Geometry: final body of the model. Coordinates: model frame, mm. A direction names the side the tool comes from. Give positions to 0.01 mm unless a question says otherwise; leave off trailing zeros. Write each loop counter-clockwise with the first axis right and the second up, starting at its lowest first coordinate (ties: lowest second). Pieces come first, ordered by that corner, then holes. Notation, with made-up numbers: (-13.75, 84) - (40.25, 84) arc R16 ccw to (40.25, 114) - close; hole circle Ø6 at (44.25, 9.25). An arc over 180 degrees is marked (long way). Use CSV: the item, a comma, the result in double quotes. Start each with the question number.
(1) Section B-B on z = -99. Output: boundary loops of the cut face in (x, y).
(2) Section D-D on y = 62. Output: boundary loops of the cut face in (x, z).
(3) Reachability of faces 1 (the flat face through (-14, -14.263, -60)), 2 (the flat face through (100, -10, 3)), 3 (the flat face through (-13, 48, -127)), 4 (the flat face through (46.2, 123.5, -39.49)) from +Z, -Z, +X, -X, +Y, -Y: full face, straight path, thin tool, end or side. Return the list, or none.
(4) Line query: probe 1 along Y at (x, z) = (-13, -113); probe 2 along X at (y, z) = (69.5, -67); probe 3 along X at (y, z) = (36, 0). Output: solid intervals per line, ascending. Write a range as [from, to].
(5) First-contact query: pin 1 Ø12 at (x, z) = (97.5, -53) entering from -Y; pin 2 Ø7.5 at (x, y) = (-12, -26.5) entering from -Z; pin 3 Ø3 at (y, z) = (55.5, -126) entering from +X. Flat tips, straight axial feed; report the tip coordinate or a pass-through.
(6) Section A-A on x = 41.5. Output: boundary loops of the cut face in (y, z).
(7) Draft query along X for faces 5 (the cylindrical face through (-13.55, 112.16, -41.09)), 6 (the flat face through (65, -10, 3)), 7 (the flat face through (-2.5, 76, -18)), 8 (the flat face through (105, -10, 3)). Return one class per face: released by +X, released by -X, zero draft, split by the parting line, or undercut.
(8) Section C-C on z = -21. Output: boundary loops of the cut face in (x, y), and give its area (3 significant figures).
from build123d import *

# Parameters (mm, degrees)
SKETCH1_W                = 170
SKETCH1_H                = 130
BOSS_EXTRUDE1_DEPTH      = 8
SKETCH2_R                = 1.5
SKETCH2_W                = 165
SKETCH2_H                = 100
CUT_EXTRUDE1_DEPTH       = 21
SKETCH3_W                = 170
SKETCH3_H                = 20
BOSS_EXTRUDE2_DEPTH      = 8
SKETCH4_W                = 65
SKETCH4_H                = 16.2
CUT_EXTRUDE2_DEPTH       = 2
SKETCH5_W                = 3.5
SKETCH5_H                = 12
CUT_EXTRUDE3_DEPTH       = 35
SKETCH6_W                = 170
SKETCH6_H                = 150
BOSS_EXTRUDE3_DEPTH      = 8
BOSS_EXTRUDE4_DEPTH      = 138
SKETCH8_W                = 249
SKETCH8_H                = 138
BOSS_EXTRUDE5_DEPTH      = 1
SKETCH9_W                = 72.8
SKETCH9_H                = 73.25
CUT_EXTRUDE4_DEPTH       = 19
BOSS_EXTRUDE6_DEPTH      = 5
SKETCH11_R               = 1.5
CUT_EXTRUDE5_DEPTH       = 56
SKETCH12_R               = 9
SKETCH12_R_2             = 6.5
SKETCH12_R_3             = 1
SKETCH12_R_4             = 2.75
CUT_EXTRUDE6_DEPTH       = 115
SKETCH13_W               = 58.59049163
SKETCH13_H               = 30.075830986
CUT_EXTRUDE7_DEPTH       = 3
FILLET1_R                = 2
SKETCH15_R               = 1.5
CUT_EXTRUDE8_DEPTH       = 10
CUT_EXTRUDE10_DEPTH      = 261
SKETCH19_R               = 1.5
BOSS_EXTRUDE7_DEPTH      = 8
BOSS_EXTRUDE12_START     = -124.5
BOSS_EXTRUDE12_DEPTH     = 249
SKETCH22_R               = 1.5
SKETCH22_W               = 165
SKETCH22_H               = 100
CUT_EXTRUDE11_DEPTH      = 18
FILLET2_R                = 10
SKETCH24_R               = 2
SKETCH24_W               = 3
SKETCH24_H               = 72
CUT_EXTRUDE15_DEPTH      = 42
CUT_EXTRUDE16_DEPTH      = 140
CUT_EXTRUDE16_DEPTH_BACK = 242
SKETCH27_W               = 249
SKETCH27_H               = 105
BOSS_EXTRUDE13_DEPTH     = 7
CUT_EXTRUDE17_DEPTH      = 249
FILLET6_R                = 3
FILLET7_R                = 3
BOSS_EXTRUDE14_DEPTH     = 9
SKETCH30_R               = 1.5
CUT_EXTRUDE18_DEPTH      = 10
SKETCH31_R               = 1.5
CUT_EXTRUDE19_DEPTH      = 49
CUT_EXTRUDE20_DEPTH      = 49
SKETCH33_W               = 129
SKETCH33_H               = 190
CUT_EXTRUDE21_DEPTH      = 200


with BuildPart() as part:
    # Sketch1 → Boss-Extrude1 (new body)
    with BuildSketch(Plane.XY):
        with Locations((85, 65)):
            Rectangle(SKETCH1_W, SKETCH1_H)
    extrude(amount=BOSS_EXTRUDE1_DEPTH)

    # Sketch2 → Cut-Extrude1 (cut)
    with BuildSketch(Plane.XY.offset(8)):
        with Locations((6.55, 123.35)):
            Circle(SKETCH2_R)
        with Locations((163.45, 123.35)):
            Circle(SKETCH2_R)
        with Locations((6.55, 6.65)):
            Circle(SKETCH2_R)
        with Locations((163.45, 6.65)):
            Circle(SKETCH2_R)
        with Locations((85, 65)):
            Rectangle(SKETCH2_W, SKETCH2_H)
    extrude(amount=-CUT_EXTRUDE1_DEPTH, mode=Mode.SUBTRACT)

    # Sketch3 → Boss-Extrude2 (add)
    with BuildSketch(Plane.XY.offset(8)):
        with Locations((85, -10)):
            Rectangle(SKETCH3_W, SKETCH3_H)
    extrude(amount=-BOSS_EXTRUDE2_DEPTH)

    # Sketch4 → Cut-Extrude2 (cut)
    with BuildSketch(Plane.XY.offset(8)):
        with Locations((85, -10)):
            Rectangle(SKETCH4_W, SKETCH4_H)
    extrude(amount=-CUT_EXTRUDE2_DEPTH, mode=Mode.SUBTRACT)

    # Sketch5 → Cut-Extrude3 (cut)
    with BuildSketch(Plane.XY.offset(6)):
        with Locations((63.25, -10)):
            Rectangle(SKETCH5_W, SKETCH5_H)
        with Locations((71.75, -10)):
            Rectangle(SKETCH5_W, SKETCH5_H)
        with Locations((80.75, -10)):
            Rectangle(SKETCH5_W, SKETCH5_H)
        with Locations((89.25, -10)):
            Rectangle(SKETCH5_W, SKETCH5_H)
        with Locations((98.25, -10)):
            Rectangle(SKETCH5_W, SKETCH5_H)
        with Locations((106.75, -10)):
            Rectangle(SKETCH5_W, SKETCH5_H)
    extrude(amount=-CUT_EXTRUDE3_DEPTH, mode=Mode.SUBTRACT)

    # Sketch6 → Boss-Extrude3 (add)
    with BuildSketch(Plane.XY.offset(8)):
        Polygon((15.504384948, 140), (225, 140), (225, -35), (-10, -35), (-10, 140), align=None)
        with Locations((85, 55)):
            Rectangle(SKETCH6_W, SKETCH6_H, mode=Mode.SUBTRACT)
    extrude(amount=-BOSS_EXTRUDE3_DEPTH)

    # Sketch7 → Boss-Extrude4 (add)
    with BuildSketch(Plane.XY.offset(8)):
        Polygon((-10, 140), (-17, 140), (-17, -42), (232, -42), (232, 140), (225, 140), (225, -35), (-10, -35), align=None)
    extrude(amount=-BOSS_EXTRUDE4_DEPTH)

    # Sketch8 → Boss-Extrude5 (add)
    with BuildSketch(Plane.XZ.offset(42)):
        with Locations((107.5, -61)):
            Rectangle(SKETCH8_W, SKETCH8_H)
    extrude(amount=BOSS_EXTRUDE5_DEPTH)

    # Sketch9 → Cut-Extrude4 (cut)
    with BuildSketch(Plane(origin=(232, 0, 0), x_dir=(0, 0, -1), z_dir=(1, 0, 0))):
        with Locations((75, 35)):
            Rectangle(SKETCH9_W, SKETCH9_H)
    extrude(amount=-CUT_EXTRUDE4_DEPTH, mode=Mode.SUBTRACT)

    # Sketch10 → Boss-Extrude6 (add)
    with BuildSketch(Plane(origin=(232, 0, 0), x_dir=(0, 0, -1), z_dir=(1, 0, 0))):
        Polygon((36, 44), (36, -4), (114, -4), (114, 44), (119, 44), (119, -9), (31, -9), (31, 44), align=None)
    extrude(amount=BOSS_EXTRUDE6_DEPTH)

    # Sketch11 → Cut-Extrude5 (cut)
    with BuildSketch(Plane(origin=(237, 0, 0), x_dir=(0, 0, -1), z_dir=(1, 0, 0))):
        with Locations((33.5, 17.5)):
            Circle(SKETCH11_R)
        with Locations((116.5, 17.5)):
            Circle(SKETCH11_R)
    extrude(amount=-CUT_EXTRUDE5_DEPTH, mode=Mode.SUBTRACT)

    # Sketch12 → Cut-Extrude6 (cut)
    with BuildSketch(Plane(origin=(0, -35, 0), x_dir=(1, 0, 0), z_dir=(0, 1, 0))):
        with Locations(Location((166.25, 32.5, 0), (0, 0, 180))):
            Circle(SKETCH12_R)
        with Locations(Location((166.25, 97.5, 0), (0, 0, 180))):
            Circle(SKETCH12_R_2)
        with Locations(Location((155.75, 97.5, 0), (0, 0, 180))):
            Circle(SKETCH12_R_3)
        with Locations(Location((155.75, 85, 0), (0, 0, 180))):
            Circle(SKETCH12_R_3)
        with Locations(Location((176.75, 85, 0), (0, 0, 180))):
            Circle(SKETCH12_R_3)
        with Locations(Location((176.75, 97.5, 0), (0, 0, 180))):
            Circle(SKETCH12_R_3)
        with Locations(Location((145.25, 97.5, 0), (0, 0, 180))):
            Circle(SKETCH12_R_4)
        with Locations(Location((187.25, 97.5, 0), (0, 0, 180))):
            Circle(SKETCH12_R_4)
    extrude(amount=-CUT_EXTRUDE6_DEPTH, mode=Mode.SUBTRACT)

    # Sketch13 → Cut-Extrude7 (cut)
    with BuildSketch(Plane.XZ.offset(43)):
        with Locations((166.25, -93.48757215)):
            Rectangle(SKETCH13_W, SKETCH13_H)
    extrude(amount=-CUT_EXTRUDE7_DEPTH, mode=Mode.SUBTRACT)

    # Fillet1
    fillet1_edges = [part.edges().sort_by_distance(p)[0] for p in [
        (136.954754185, -40, -93.48757215),
        (166.25, -40, -78.449656657),
        (195.545245815, -40, -93.48757215),
        (166.25, -40, -108.525487643),
    ]]
    fillet(fillet1_edges, radius=FILLET1_R)

    # Sketch15 → Cut-Extrude8 (cut)
    with BuildSketch(Plane(origin=(0, 140, 0), x_dir=(1, 0, 0), z_dir=(0, 1, 0))):
        with Locations(Location((5, -4, 0), (0, 0, 270))):
            Circle(SKETCH15_R)
        with Locations(Location((20, -4, 0), (0, 0, 270))):
            Circle(SKETCH15_R)
        with Locations(Location((217, -4, 0), (0, 0, 90))):
            Circle(SKETCH15_R)
        with Locations(Location((202, -4, 0), (0, 0, 90))):
            Circle(SKETCH15_R)
    extrude(amount=-CUT_EXTRUDE8_DEPTH, mode=Mode.SUBTRACT)

    # Sketch18 → Cut-Extrude10 (cut)
    with BuildSketch(Plane(origin=(232, 0, 0), x_dir=(0, 0, -1), z_dir=(1, 0, 0))):
        Polygon((45.496279283, 140), (-8, 140), (-8, 15), (0, 15), align=None)
    extrude(amount=-CUT_EXTRUDE10_DEPTH, mode=Mode.SUBTRACT)

    # Sketch19 → Boss-Extrude7 (add)
    with BuildSketch(Plane.XY.offset(8)):
        with Locations((6.55, 6.65)):
            Circle(SKETCH19_R)
        with Locations((163.45, 6.65)):
            Circle(SKETCH19_R)
    extrude(amount=-BOSS_EXTRUDE7_DEPTH)

    # Sketch21 → Boss-Extrude12 (add)
    with BuildSketch(Plane(origin=(107.5, 0, 0), x_dir=(0, 0, -1), z_dir=(1, 0, 0)).offset(BOSS_EXTRUDE12_START)):
        Polygon((45.496279283, 140), (0, 15), (-8, 15), (37.496279283, 140), align=None)
    extrude(amount=BOSS_EXTRUDE12_DEPTH)

    # Sketch22 → Cut-Extrude11 (cut)
    with BuildSketch(Plane(origin=(0, 4.325817115, 11.885084845), x_dir=(1, 0, 0), z_dir=(0, 0.3420201433256603, 0.9396926207859115))):
        with Locations(Location((1.55, 136.220338945, 0), (0, 0, 270))):
            Circle(SKETCH22_R)
        with Locations(Location((158.45, 136.220338945, 0), (0, 0, 270))):
            Circle(SKETCH22_R)
        with Locations(Location((1.55, 19.520338945, 0), (0, 0, 270))):
            Circle(SKETCH22_R)
        with Locations(Location((158.45, 19.520338945, 0), (0, 0, 270))):
            Circle(SKETCH22_R)
        with Locations((80, 77.870338945)):
            Rectangle(SKETCH22_W, SKETCH22_H)
    extrude(amount=-CUT_EXTRUDE11_DEPTH, mode=Mode.SUBTRACT)

    # Fillet2
    fillet2_edges = [part.edges().sort_by_distance(p)[0] for p in [
        (107.5, 15, 8),
    ]]
    fillet(fillet2_edges, radius=FILLET2_R)

    # Sketch24 → Cut-Extrude15 (cut)
    with BuildSketch(Plane(origin=(-10, 0, 0), x_dir=(0, 0, -1), z_dir=(1, 0, 0))):
        with Locations(Location((113.5, 48.5, 0), (0, 0, 90))):
            Circle(SKETCH24_R)
        with Locations(Location((119.5, 68.5, 0), (0, 0, 90))):
            Circle(SKETCH24_R)
        with Locations(Location((119.5, 28.5, 0), (0, 0, 90))):
            Circle(SKETCH24_R)
        with Locations((128.5, 48.5)):
            Rectangle(SKETCH24_W, SKETCH24_H)
    extrude(amount=-CUT_EXTRUDE15_DEPTH, mode=Mode.SUBTRACT)

    # Sketch25 → Cut-Extrude16 (cut, two sides: drawn at the far end of the back side and taken through both)
    with BuildSketch(Plane(origin=(232, 0, 0), x_dir=(0, 0, -1), z_dir=(1, 0, 0)).offset(-CUT_EXTRUDE16_DEPTH_BACK)):
        Polygon((45.496279283, 140), (130, 140), (130, -43), (0, -43), (0, 15), align=None)
    extrude(amount=CUT_EXTRUDE16_DEPTH + CUT_EXTRUDE16_DEPTH_BACK, mode=Mode.SUBTRACT)

    # Sketch27 → Boss-Extrude13 (add)
    with BuildSketch(Plane(origin=(0, 140, 0), x_dir=(1, 0, 0), z_dir=(0, 1, 0))):
        with Locations((107.5, 89.996279283)):
            Rectangle(SKETCH27_W, SKETCH27_H)
    extrude(amount=BOSS_EXTRUDE13_DEPTH)

    # Sketch28 → Cut-Extrude17 (cut)
    with BuildSketch(Plane(origin=(232, 0, 0), x_dir=(0, 0, -1), z_dir=(1, 0, 0))):
        Polygon((37.496279283, 140), (40.044070923, 147), (37.496279283, 147), align=None)
    extrude(amount=-CUT_EXTRUDE17_DEPTH, mode=Mode.SUBTRACT)

    # Fillet6
    fillet6_edges = [part.edges().sort_by_distance(p)[0] for p in [
        (107.5, 140, -142.496279283),
    ]]
    fillet(fillet6_edges, radius=FILLET6_R)

    # Fillet7
    fillet7_edges = [part.edges().sort_by_distance(p)[0] for p in [
        (-17, 145, -142.496279283),
        (-17, 140, -134.748139642),
        (-17, 140.878679656, -141.617599627),
    ]]
    fillet(fillet7_edges, radius=FILLET7_R)

    # Sketch29 → Boss-Extrude14 (add)
    with BuildSketch(Plane(origin=(232, 0, 0), x_dir=(0, 0, -1), z_dir=(1, 0, 0))):
        with BuildLine():
            Line((-8, -43), (0, -43))
            Line((0, -43), (0, 15))
            Line((0, 15), (45.496279283, 140))
            Line((45.496279283, 140), (139.496279283, 140))
            ThreePointArc((139.496279283, 140), (141.886652657, 140.990125071), (142.876777727, 143.380498444))
            Line((142.876777727, 143.380498444), (142.496279283, 147))
            Line((142.496279283, 147), (40.044070923, 147))
            Line((40.044070923, 147), (-7.396926208, 16.656931626))
            ThreePointArc((-7.396926208, 16.656931626), (-7.84807753, 14.97321197), (-8, 13.236730193))
            Line((-8, 13.236730193), (-8, -43))
        make_face()
    extrude(amount=BOSS_EXTRUDE14_DEPTH)

    # Sketch30 → Cut-Extrude18 (cut)
    with BuildSketch(Plane(origin=(0, 147, 0), x_dir=(1, 0, 0), z_dir=(0, 1, 0))):
        with Locations(Location((218.25, 136.876777727, 0), (0, 0, 270))):
            Circle(SKETCH30_R)
        with Locations(Location((203.25, 136.876777727, 0), (0, 0, 270))):
            Circle(SKETCH30_R)
    extrude(amount=-CUT_EXTRUDE18_DEPTH, mode=Mode.SUBTRACT)

    # Sketch31 → Cut-Extrude19 (cut)
    with BuildSketch(Plane.XY.offset(8)):
        with Locations((219, -39)):
            Circle(SKETCH31_R)
        with Locations((204, -39)):
            Circle(SKETCH31_R)
    extrude(amount=-CUT_EXTRUDE19_DEPTH, mode=Mode.SUBTRACT)

    # Sketch32 → Cut-Extrude20 (cut)
    with BuildSketch(Plane.ZY.offset(17)):
        with BuildLine():
            Line((-110, 0.736730193), (-12, 0.736730193))
            ThreePointArc((-12, 0.736730193), (-4.5, -6.763269807), (-12, -14.263269807))
            Line((-12, -14.263269807), (-110, -14.263269807))
            ThreePointArc((-110, -14.263269807), (-117.5, -6.763269807), (-110, 0.736730193))
        make_face()
        with BuildLine():
            Line((-110, 119.5), (-48.588668173, 119.5))
            ThreePointArc((-48.588668173, 119.5), (-41.088668173, 112), (-48.588668173, 104.5))
            Line((-48.588668173, 104.5), (-110, 104.5))
            ThreePointArc((-110, 104.5), (-117.5, 112), (-110, 119.5))
        make_face()
    extrude(amount=-CUT_EXTRUDE20_DEPTH, mode=Mode.SUBTRACT)

    # Sketch33 → Cut-Extrude21 (cut)
    with BuildSketch(Plane.XY.offset(8)):
        with Locations((176.5, 52)):
            Rectangle(SKETCH33_W, SKETCH33_H)
    extrude(amount=-CUT_EXTRUDE21_DEPTH, mode=Mode.SUBTRACT)


solid = part.part
Check values:
1,outline,"(-17, -43) - (-10, -43) - (-10, -14.26) - (-17, -14.26) - close; (-17, 0.74) - (-10, 0.74) - (-10, 104.5) - (-17, 104.5) - close; (-17, 119.5) - (-10, 119.5) - (-10, 140) - (112, 140) - (112, 147) - (-17, 147) - close"
2,outline,"(-17, -127) - (-10, -127) - (-10, -17.11) - (-2.5, -17.11) - (-2.5, -9.11) - (-17, -9.11) - close"
3,face 1,"+X, -X"
3,face 2,"+Z, -Z"
3,face 3,"-Z, +X, -X"
3,face 4,"-Z, +X, -Y"
4,probe 1,"y = [-43, -13.64], [0.11, 46.56], [50.44, 105.13], [118.87, 147]"
4,probe 2,"x = [-17, -10]"
4,probe 3,"x = [-17, -2.5]"
5,pin 1,"stops at y = 140"
5,pin 2,"stops at z = -130"
5,pin 3,"stops at x = -10"
6,outline,"(-43, 0) - (15, 0) - (27.94, -4.71) - (30.52, 2.35) - (16.66, 7.4) arc R10 ccw to (13.24, 8) - (-43, 8) - close; (121.91, -38.91) - (140, -45.5) - (140, -139.5) arc R3 ccw to (143, -142.5) - (147, -142.5) - (147, -40.04) - (124.48, -31.85) - close"
7,face 5,"zero draft"
7,face 6,"undercut"
7,face 7,"released by +X"
7,face 8,"undercut"
8,outline,"(-17, -43) - (-10, -43) - (-10, -14.26) - (-17, -14.26) - close; (-17, 0.74) - (-10, 0.74) - (-10, 72.7) - (-2.5, 72.7) - (-2.5, 94.68) - (-17, 94.68) - close"
8,area,"1,020 mm²"
